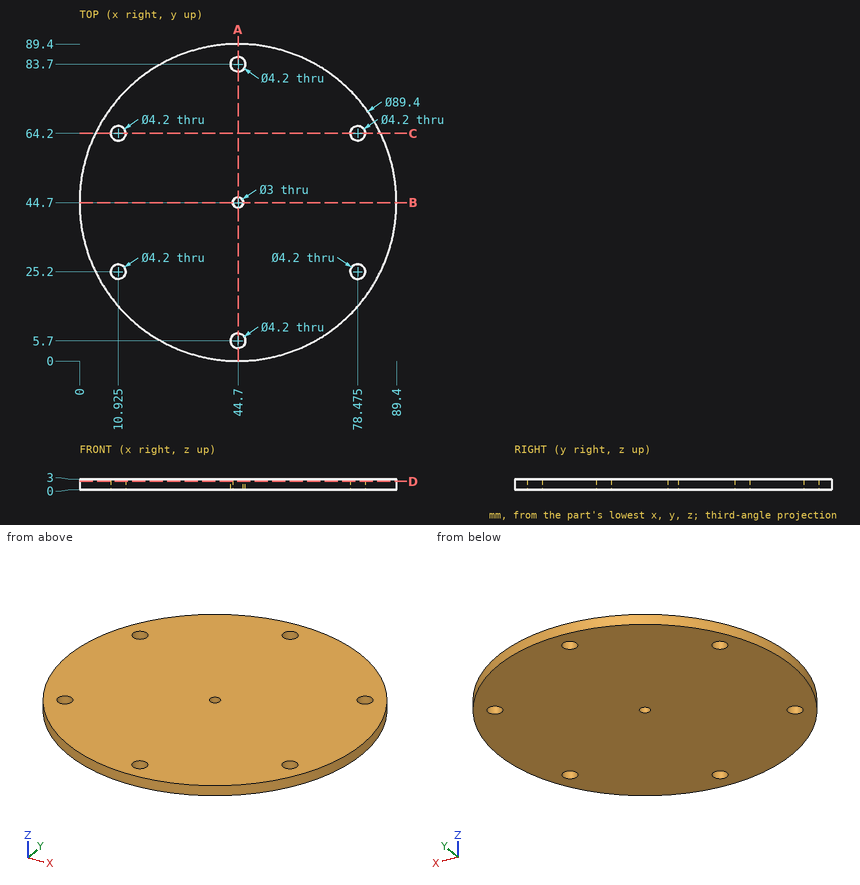
Could you check a few things on this drawing? It's one solid part, dimensions in mm from its lowest x, y, z. Coordinates: 2 decimals unless noted, no trailing zeros. Order: outer loops, then holes, each group sorted by start corner. A loop starts at its lowest first (then second) coordinate and runs counter-clockwise, first axis right, second up.
1) I need wall thicknesses on line 1 (Y direction, x = 44.7, z = 1.9); line 2 (X direction, y = 64.2, z = 1.55) (3 decimals); line 3 (Y direction, x = 77, z = 1.75). Which ranges of each line are inside material? Lowest first, please.
2) Will these pins go through, and if not, where does the flat tip stop? pin 1 (2.5 mm diameter, centred on x = 10.93, y = 25.2, fed in from -Z); pin 2 (5 mm diameter, centred on x = 44.7, y = 44.7, fed in from -Z); pin 3 (1 mm diameter, centred on y = 69, z = 1, fed in from +X); pin 4 (1 mm diameter, centred on x = 31, z = 2.5, fed in from +Y).
3) Imagine slicing it at A-A on x = 44.7. List the corners of the cut face in (y, z) for me, and give its area (3 significant figures).
4) Imagine slicing it at D-D on z = 2.35. List the corners of the cut face in (x, y) for me (3 decimals), and give its area (3 significant figures).
5) Imagine slicing it at B-B on y = 44.7. List the corners of the cut face in (x, z) for me.
6) Imagine slicing it at C-C on y = 64.2. List the corners of the cut face in (x, z) for me (3 decimals).
Response values:
1. line 1: y = 0 to 3.6, 7.8 to 43.2, 46.2 to 81.6, 85.8 to 89.4
1. line 2: x = 4.478 to 8.825, 13.025 to 76.375, 80.575 to 84.922
1. line 3: y = 13.8 to 23.71, 26.69 to 62.71, 65.69 to 75.6
2. pin 1: passes through
2. pin 2: stops at z = 0
2. pin 3: stops at x = 82.54
2. pin 4: stops at y = 87.41
3. outline: (0, 0) - (3.6, 0) - (3.6, 3) - (0, 3) - close; (7.8, 0) - (43.2, 0) - (43.2, 3) - (7.8, 3) - close; (46.2, 0) - (81.6, 0) - (81.6, 3) - (46.2, 3) - close; (85.8, 0) - (89.4, 0) - (89.4, 3) - (85.8, 3) - close
3. area: 234 mm2
4. outline: circle Ø89.4 at (44.7, 44.7); hole circle Ø4.2 at (10.925, 25.2); hole circle Ø4.2 at (10.925, 64.2); hole circle Ø4.2 at (44.7, 5.7); hole circle Ø4.2 at (44.7, 83.7); hole circle Ø3 at (44.7, 44.7); hole circle Ø4.2 at (78.475, 25.2); hole circle Ø4.2 at (78.475, 64.2)
4. area: 6,190 mm2
5. outline: (0, 0) - (43.2, 0) - (43.2, 3) - (0, 3) - close; (46.2, 0) - (89.4, 0) - (89.4, 3) - (46.2, 3) - close
6. outline: (4.478, 0) - (8.825, 0) - (8.825, 3) - (4.478, 3) - close; (13.025, 0) - (76.375, 0) - (76.375, 3) - (13.025, 3) - close; (80.575, 0) - (84.922, 0) - (84.922, 3) - (80.575, 3) - close
